```python
from build123d import *

# Parameters (mm, degrees)
SKETCH1_W                    = 15
SKETCH1_H                    = 24
BOSS_EXTRUDE1_DEPTH          = 6
SKETCH2_R                    = 5.25
CUT_EXTRUDE1_DEPTH           = 3.5
CUT_EXTRUDE2_REACH           = 24.136
CUT_EXTRUDE2_END_RADIUS      = 5.25
SKETCH3_W                    = 3.5
SKETCH3_H                    = 3.2
SKETCH4_W                    = 7
SKETCH4_H                    = 2
CUT_EXTRUDE3_DEPTH           = 10
SKETCH5_R                    = 0.8
CUT_EXTRUDE4_DEPTH           = 1.2
SKETCH6_OUTSIDE_W            = 22.786
SKETCH6_OUTSIDE_H            = 31.786
SKETCH6_OUTSIDE_R            = 6
CUT_EXTRUDE5_DEPTH           = 4
M2_5X0_45_TAPPED_HOLE1_D     = 2.05
M2_5X0_45_TAPPED_HOLE1_DEPTH = 6.35
M2_5X0_45_TAPPED_HOLE1_TIP   = 0.615882135
FILLET1_R                    = 1


with BuildPart() as part:
    # Sketch1 → Boss-Extrude1 (new body)
    with BuildSketch(Plane(origin=(0, 0, -7.5), x_dir=(0, 0, 1), z_dir=(-1, 0, 0))):
        Rectangle(SKETCH1_W, SKETCH1_H)
    extrude(amount=BOSS_EXTRUDE1_DEPTH)

    # Sketch2 → Cut-Extrude1 (cut)
    with BuildSketch(Plane.ZY.offset(6)):
        with Locations((-7.5, 0)):
            Circle(SKETCH2_R)
    extrude(amount=-CUT_EXTRUDE1_DEPTH, mode=Mode.SUBTRACT)

    # Cut-Extrude2: up to this cylinder (the profile starts outside it)
    cut_extrude2_end = Plane(origin=(-4.25, 0, -7.5), z_dir=(-1, 0, 0)) * Cylinder(CUT_EXTRUDE2_END_RADIUS, 59.772, mode=Mode.PRIVATE)
    # Sketch3 → Cut-Extrude2 (cut, up to the surface)
    with BuildSketch(Plane(origin=(5, 0, 0), x_dir=(1, 0, 0), z_dir=(0, 0, 1)), mode=Mode.PRIVATE) as cut_extrude2_sk1:
        with Locations((-9.25, 0)):
            Rectangle(SKETCH3_W, SKETCH3_H)
    cut_extrude2_tool1 = extrude(cut_extrude2_sk1.sketch, amount=-CUT_EXTRUDE2_REACH, mode=Mode.PRIVATE) - cut_extrude2_end
    add(cut_extrude2_tool1.solids().sort_by_distance((-4.25, 0, 0))[0], mode=Mode.SUBTRACT)

    # Sketch4 → Cut-Extrude3 (cut)
    with BuildSketch(Plane(origin=(0, 0, 0), x_dir=(0, 0, -1), z_dir=(1, 0, 0))):
        with Locations((7.5, 9)):
            Rectangle(SKETCH4_W, SKETCH4_H)
        with Locations((7.5, -9)):
            Rectangle(SKETCH4_W, SKETCH4_H)
    extrude(amount=-CUT_EXTRUDE3_DEPTH, mode=Mode.SUBTRACT)

    # Sketch5 → Cut-Extrude4 (cut)
    with BuildSketch(Plane.ZY.offset(2.5)):
        with Locations((-7.5, 0)):
            Circle(SKETCH5_R)
    extrude(amount=-CUT_EXTRUDE4_DEPTH, mode=Mode.SUBTRACT)

    # Sketch6 outside → Cut-Extrude5 (cut)
    with BuildSketch(Plane(origin=(0, 0, 0), x_dir=(0, 0, -1), z_dir=(1, 0, 0))):
        with Locations((7.5, 0)):
            Rectangle(SKETCH6_OUTSIDE_W, SKETCH6_OUTSIDE_H)
        with Locations((7.5, 0)):
            Circle(SKETCH6_OUTSIDE_R, mode=Mode.SUBTRACT)
    extrude(amount=-CUT_EXTRUDE5_DEPTH, mode=Mode.SUBTRACT)

    # M2.5x0.45 Tapped Hole1
    with Locations(Plane.ZY.offset(6)):
        with Locations((-12.5, 6.5), (-2.5, 6.5), (-2.5, -6.5), (-12.5, -6.5)):
            Hole(M2_5X0_45_TAPPED_HOLE1_D / 2, depth=M2_5X0_45_TAPPED_HOLE1_DEPTH)
            with Locations((0, 0, -(M2_5X0_45_TAPPED_HOLE1_DEPTH + M2_5X0_45_TAPPED_HOLE1_TIP / 2))):  # 118° drill point
                Cone(0, M2_5X0_45_TAPPED_HOLE1_D / 2, M2_5X0_45_TAPPED_HOLE1_TIP, mode=Mode.SUBTRACT)

    # Fillet1
    fillet1_edges = [part.edges().sort_by_distance(p)[0] for p in [
        (0, 0, -1.5),
        (-4, -12, -7.5),
        (-4, 12, -7.5),
    ]]
    fillet(fillet1_edges, radius=FILLET1_R)


solid = part.part
```
Geometry: final body of the model. Coordinates: model frame, mm. A direction names the side the tool comes from. Give positions to 0.01 mm unless a question says otherwise; leave off trailing zeros. Order: outer loops, then holes, each group sorted by start corner. A loop starts at its lowest first (then second) coordinate and runs counter-clockwise, first axis right, second up. Notation, with made-up numbers: (60.25, 31.25) -> (67.25, 31.25) arc R18 ccw to (67.25, 45.25) -> close; hole circle Ø11 at (59, 57). An arc over 180 degrees is marked (long way). Write each question's results on one line, items separated by ' | '. Start each with the question number.
1) First-contact query: pin 1 (1 mm diameter, centred on x = -4.5, z = -7.5, fed in from -Y); pin 2 (5 mm diameter, centred on y = -1.5, z = -6.5, fed in from -X); pin 3 (1.5 mm diameter, centred on x = -1.5, z = -4, fed in from -Y). Flat tips, straight axial feed; report the tip coordinate or a pass-through.
2) Set-up query: faces 1 (the cylindrical face through (-1.9, 0, -8.3)), 2 (the flat face through (-5, 8, -7)), 3 (the flat face through (-5, 1.6, -2)), 4 (the flat face through (-5, -7, 0)), 5 (the flat face through (-4, 0, -14)). Return all of +Z, -Z, +X, -X, +Y, -Y with unobstructed straight access to the full face (end or side cutting, diameter ignored); none if empty.
3) Section D-D (x = -2.05). Return loops of the section in (y, z), then the cut area to 3 significant figures.
4) Draft query along Z for faces 6 (the flat face through (-5, 0, -15)), 7 (the flat face through (-5, -1.6, -2)), 8 (the flat face through (-5, 10, -7)). Return one class per face: pulls with the +Z half, pulls with the -Z half, needs draft (parallel to the pull), parting line crosses it, or undercut.
5) Section C-C (z = -7.5). Return loops of the section in (x, y).
6) Section B-B (x = -5.55). Return loops of the section in (y, z) (3 decimals).
7) Line query: line 1 (Y direction, x = -4.15, z = -9.25); line 2 (Y direction, x = -2.1, z = -7.5); line 3 (X direction, y = -8, z = -14). Output: solid intervals per line, ascending. Write a range as from..to.
8) Section A-A (y = 6.5). Return loops of the section in (x, z) (3 decimals), then the cut area to 3 significant figures.
Calculated:
1) pin 1: y = -12 | pin 2: x = -2.5 | pin 3: y = -5.33
2) face 1: -X | face 2: +X, -X | face 3: +Z, -X | face 4: +Z, +X, -X, +Y, -Y | face 5: +X
3) outline: circle Ø12 at (0, -7.5); hole circle Ø1.6 at (0, -7.5) | area: 111 mm2
4) face 6: pulls with the -Z half | face 7: needs draft | face 8: undercut
5) outline: (-6, -12) -> (-5, -12) arc R1 ccw to (-4, -11) -> (-4, -10) -> (-6, -10) -> close; (-6, -8) -> (-4, -8) -> (-4, -6) -> (-1, -6) arc R1 ccw to (0, -5) -> (0, 5) arc R1 ccw to (-1, 6) -> (-4, 6) -> (-4, 8) -> (-6, 8) -> (-6, 5.25) -> (-2.5, 5.25) -> (-2.5, 0.8) -> (-1.3, 0.8) -> (-1.3, -0.8) -> (-2.5, -0.8) -> (-2.5, -5.25) -> (-6, -5.25) -> close; (-6, 10) -> (-4, 10) -> (-4, 11) arc R1 ccw to (-5, 12) -> (-6, 12) -> close
6) outline: (-12, -15) -> (12, -15) -> (12, 0) -> (1.6, 0) -> (1.6, -2.5) arc R5.25 cw (long way) to (-1.6, -2.5) -> (-1.6, 0) -> (-12, 0) -> close; hole (-10, -11) -> (-8, -11) -> (-8, -4) -> (-10, -4) -> close; hole circle Ø2.05 at (-6.5, -12.5); hole circle Ø2.05 at (-6.5, -2.5); hole circle Ø2.05 at (6.5, -12.5); hole circle Ø2.05 at (6.5, -2.5); hole (8, -11) -> (10, -11) -> (10, -4) -> (8, -4) -> close
7) line 1: -11.53..-10, -8..-4.95, 4.95..8, 10..11.53 | line 2: -6..-0.8, 0.8..6 | line 3: -6..-4
8) outline: (-6, -15) -> (-4, -15) -> (-4, -13.525) -> (-6, -13.525) -> close; (-6, -11.475) -> (-4, -11.475) -> (-4, -3.525) -> (-6, -3.525) -> close; (-6, -1.475) -> (-4, -1.475) -> (-4, 0) -> (-6, 0) -> close | area: 21.8 mm2
